```python
from build123d import *

# Parameters (mm, degrees)
F1_DEPTH = 40
F2_SIZE  = 1.5


with BuildPart() as f1:
    # F0 (on Front) → F1 (new body)
    with BuildSketch(Plane.XZ):
        with BuildLine():
            Line((11.307107, 6.555), (8.768918, 4.016812))
            Line((8.768918, 4.016812), (18, 4.016812))
            Line((18, 4.016812), (17.5, 6.516812))
            Line((17.5, 6.516812), (20, 7.016812))
            ThreePointArc((20, 7.016812), (0, 13.293998), (-20, 7.016812))
            Line((-20, 7.016812), (-17.5, 6.516812))
            Line((-17.5, 6.516812), (-18, 4.016812))
            Line((-18, 4.016812), (-8.768918, 4.016812))
            Line((-8.768918, 4.016812), (-11.307107, 6.555))
            Line((-11.307107, 6.555), (-8.091484, 9.770623))
            ThreePointArc((-8.091484, 9.770623), (0, 10.793998), (8.091484, 9.770623))
            Line((8.091484, 9.770623), (11.307107, 6.555))
        make_face()
    extrude(amount=-F1_DEPTH)

    # F2
    f2_edges = [f1.edges().sort_by_distance(p)[0] for p in [
        (0, 0, 13.293998),
        (0, 40, 13.293998),
    ]]
    chamfer(f2_edges, length=F2_SIZE)


solid = f1.part
```
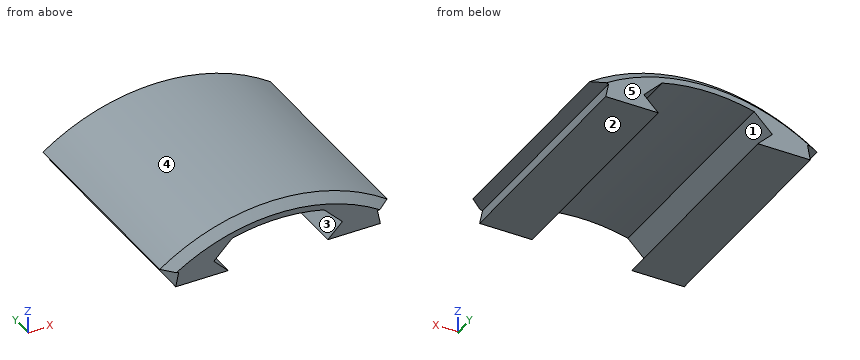
For this review, take the finished solid that the model builds, in its own axes (mm). Face numbers are marked on the shaded views. A direction names the side the tool comes from. Coordinates: 2 decimals unless noted, no trailing zeros. Loops run counter-clockwise (first coordinate to the right, second up) from the corner with the lowest first, then second, coordinate; pieces in that order, holes last. Notation, with made-up numbers: (-14, -23) - (-8, -23) arc R10 ccw to (-8, -18) - close; hole circle Ø11 at (64.25, 79.25). An arc over 180 degrees is marked (long way). Use one line per item in the form item = value. Start each with the question number.
1) For the marked faces 1 and 2, list the 3-axis set-ups (+Z, -Z, +X, -X, +Y, -Y) from which the entire face can be reached by the end or side of a thin tool; tool diameter is ignored.
2) Draft analysis for pull direction X (two halves, no side actions). For the marked faces 3, 4 and 5, state which applies: released by +X, released by -X, zero draft, split by the parting line, or undercut.
3) Take a section at A-A (y = 3). State the section outline as (x, z) points (3 decimals).
4) For pin 1 (2 mm diameter, centred on x = 12.5, y = 12, fed in from +Z); pin 2 (4 mm diameter, centred on x = 5, y = 11, fed in from -Z); pin 3 (4 mm diameter, centred on x = -7, z = 6.5, fed in from -Y); pin 4 (2 mm diameter, centred on y = 4.5, z = 11, fed in from +X), all flat-tipped, find the tip position at first contact; note any pin that passes through.
5) To check wall thickness, follow probe 1 along Z at (x, y) = (13, 37); probe 2 along X at (y, z) = (21.5, 7.5); probe 3 along Z at (x, y) = (0.5, 34). State the ranges of each line that lie inside material, in increasing order. Write a range as from..to.
From the geometry:
q1.face_1 = +Y, -Y
q1.face_2 = -Z, +X, -X, +Y, -Y
q2.face_3 = undercut
q2.face_4 = split by the parting line
q2.face_5 = zero draft
q3.outline = (-20, 7.017) - (-17.5, 6.517) - (-18, 4.017) - (-8.769, 4.017) - (-11.307, 6.555) - (-8.091, 9.771) arc R32.5 cw to (8.091, 9.771) - (11.307, 6.555) - (8.769, 4.017) - (18, 4.017) - (17.5, 6.517) - (20, 7.017) arc R35 ccw to start
q4.pin_1 = 11.35
q4.pin_2 = 10.03
q4.pin_3 = through
q4.pin_4 = 14.82
q5.probe_1 = 4.02..10.79
q5.probe_2 = -19.29..-10.36, 10.36..19.29
q5.probe_3 = 10.79..13.29
